Input: part model. Units: mm. Frame: model coordinates. A direction names the side the tool comes from. Give positions to 0.01 mm unless a question says otherwise; leave off trailing zeros. Loops run counter-clockwise (first coordinate to the right, second up) from the corner with the lowest first, then second, coordinate; pieces in that order, holes last.
from build123d import *

# Parameters (mm, degrees)
F1_R     = 57.15
F1_R_2   = 50.8
F3_DEPTH = 812.8
F4_DEPTH = 800.1


with BuildPart() as f2:
    # F2: sweep along a path in F0
    with BuildLine(Plane.XZ) as f2_path:
        Line((0, 0), (152.4, 0))
        ThreePointArc((152.4, 0), (260.1630734528, 44.6369265472), (304.8, 152.4))
        Line((304.8, 152.4), (304.8, 304.8))
    # F1 (on Right) → F2 (sweep)
    with BuildSketch(Plane.YZ):
        Circle(F1_R)
        Circle(F1_R_2, mode=Mode.SUBTRACT)
    sweep(path=f2_path.line)

    # F3 (add): a face of the model
    f3_faces = [f2.faces().sort_by_distance(p)[0] for p in [
        (304.8, -55.5335538982, 304.8),
    ]]
    extrude(f3_faces, amount=F3_DEPTH)

    # F4 (add): a face of the model
    f4_faces = [f2.faces().sort_by_distance(p)[0] for p in [
        (0, -55.5335538982, 0),
    ]]
    extrude(f4_faces, amount=F4_DEPTH)


solid = f2.part
(1) Cut plane C-C (z = 957). Return the cut outline in (x, y).
Values follow:
outline: circle Ø114.3 at (304.8, 0); hole circle Ø101.6 at (304.8, 0)
(2) Pin query (flat end, axial travel): pin 1 Ø4 at (x, y) = (-81.5, 20.5) entering from -Z; pin 2 Ø1.5 at (x, y) = (-553, 9.5) entering from -Z; pin 3 Ø6 at (y, z) = (-29.5, 669) entering from +X. Return the tip coordinate at first contact, or that it passes through.
Values follow:
pin 1: stops at z = -54.07
pin 2: stops at z = -56.48
pin 3: stops at x = 355.43
(3) Mould query, pull axis Z, two halves, no side actions, for faces 3 (the cylindrical face through (-317.182, -11.012, -49.592)), 4 (the flat face through (-800.1, 34, -38)), 5 (the cylindrical face through (-317.182, -57.095, 2.513)). Classes: +Z half, -Z half, draft (parallel to the pull), parting line (faces both ways), or undercut.
Values follow:
face 3: undercut
face 4: draft
face 5: parting line
(4) Reachability of faces 1 (the cylindrical face through (360.59, -12.39, 628.24)), 2 (the flat face through (266, -34, 1117.6)) from +Z, -Z, +X, -X, +Y, -Y: full face, straight path, thin tool, end or side. Return the list, or none.
Values follow:
face 1: +Z
face 2: +Z, +X, -X, +Y, -Y
(5) Cut plane A-A (y = 0). Return the cut outline in (x, z), and give its area (3 significant figures).
Values follow:
outline: (-800.1, -57.15) - (152.4, -57.15) arc R209.55 ccw to (361.95, 152.4) - (361.95, 1117.6) - (355.6, 1117.6) - (355.6, 152.4) arc R203.2 cw to (152.4, -50.8) - (-800.1, -50.8) - close; (-800.1, 50.8) - (152.4, 50.8) arc R101.6 ccw to (254, 152.4) - (254, 1117.6) - (247.65, 1117.6) - (247.65, 152.4) arc R95.25 cw to (152.4, 57.15) - (-800.1, 57.15) - close
area: 27,400 mm2
(6) Ray query, probe 1 along X at (y, z) = (0, 260.5); probe 2 along Z at (x, y) = (-351.5, 0). Return the intervals inside material, ascending.
Values follow:
probe 1: x = 247.65 to 254, 355.6 to 361.95
probe 2: z = -57.15 to -50.8, 50.8 to 57.15
(7) Cut plane B-B (x = -541). Return the cut outline in (y, z).
Values follow:
outline: circle Ø114.3 at (0, 0); hole circle Ø101.6 at (0, 0)
